The listing builds one solid part. Answer for the finished solid, in the listing's coordinates (mm). A direction names the side the tool comes from. Give positions to 0.01 mm unless a question says otherwise; leave off trailing zeros. Write each loop counter-clockwise with the first axis right and the second up, starting at its lowest first coordinate (ties: lowest second). Pieces come first, ordered by that corner, then holes. Notation, with made-up numbers: (-3.5, -20) - (9.5, -20) arc R28 ccw to (9.5, 16) - close; hole circle Ø5 at (31, 57.5). An arc over 180 degrees is marked (long way). Answer in a Markdown table with one row per item. Add a question column.
from build123d import *

# Parameters (mm, degrees)
SKIZZE1_W                       = 100
SKIZZE1_H                       = 50
AUFSATZ_LINEAR_AUSTRAGEN2_DEPTH = 25
SKIZZE4_R                       = 10
SCHNITT_LINEAR_AUSTRAGEN3_DEPTH = 115.564392374
SKIZZE5_W                       = 90
SKIZZE5_H                       = 40
SCHNITT_LINEAR_AUSTRAGEN4_DEPTH = 10
SKIZZE7_W                       = 25
SKIZZE7_H                       = 40
SCHNITT_LINEAR_AUSTRAGEN5_DEPTH = 10
VERRUNDUNG1_R                   = 10
VERRUNDUNG2_R                   = 10
SKIZZE8_W                       = 2
SKIZZE8_H                       = 40
SCHNITT_LINEAR_AUSTRAGEN6_DEPTH = 10
VERRUNDUNG3_R                   = 10


with BuildPart() as part:
    # Skizze1 → Aufsatz-Linear austragen2 (new body)
    with BuildSketch(Plane.XY):
        with Locations((50, 25)):
            Rectangle(SKIZZE1_W, SKIZZE1_H)
    extrude(amount=AUFSATZ_LINEAR_AUSTRAGEN2_DEPTH)

    # Skizze4 → Schnitt-Linear austragen3 (cut, through all)
    with BuildSketch(Plane(origin=(0, 50, 0), x_dir=(1, 0, 0), z_dir=(0, 1, 0))):
        with Locations((20, -25)):
            Circle(SKIZZE4_R)
        with Locations((80, -25)):
            Circle(SKIZZE4_R)
    extrude(amount=-SCHNITT_LINEAR_AUSTRAGEN3_DEPTH, mode=Mode.SUBTRACT)

    # Skizze5 → Schnitt-Linear austragen4 (cut)
    with BuildSketch(Plane(origin=(0, 0, 0), x_dir=(-1, 0, 0), z_dir=(0, 0, -1))):
        with Locations((-50, 25)):
            Rectangle(SKIZZE5_W, SKIZZE5_H)
    extrude(amount=-SCHNITT_LINEAR_AUSTRAGEN4_DEPTH, mode=Mode.SUBTRACT)

    # Skizze7 → Schnitt-Linear austragen5 (cut)
    with BuildSketch(Plane(origin=(0, 0, 10), x_dir=(-1, 0, 0), z_dir=(0, 0, -1))):
        with Locations((-50, 25)):
            Rectangle(SKIZZE7_W, SKIZZE7_H)
    extrude(amount=-SCHNITT_LINEAR_AUSTRAGEN5_DEPTH, mode=Mode.SUBTRACT)

    # Verrundung1
    verrundung1_edges = [part.edges().sort_by_distance(p)[0] for p in [
        (37.5, 25, 10),
    ]]
    fillet(verrundung1_edges, radius=VERRUNDUNG1_R - 0.0001)  # a hair under: the kernel refuses the full size

    # Verrundung2
    verrundung2_edges = [part.edges().sort_by_distance(p)[0] for p in [
        (62.5, 25, 10),
    ]]
    fillet(verrundung2_edges, radius=VERRUNDUNG2_R - 0.0001)  # a hair under: the kernel refuses the full size

    # Skizze8 → Schnitt-Linear austragen6 (cut)
    with BuildSketch(Plane(origin=(0, 0, 10), x_dir=(-1, 0, 0), z_dir=(0, 0, -1))):
        with Locations((-94, 25)):
            Rectangle(SKIZZE8_W, SKIZZE8_H)
    extrude(amount=-SCHNITT_LINEAR_AUSTRAGEN6_DEPTH, mode=Mode.SUBTRACT)

    # Verrundung3
    verrundung3_edges = [part.edges().sort_by_distance(p)[0] for p in [
        (93, 25, 10),
    ]]
    fillet(verrundung3_edges, radius=VERRUNDUNG3_R - 0.0001)  # a hair under: the kernel refuses the full size


solid = part.part
1. Straight lines are drawn through the part: L1, parallel to X at y = 8, z = 9.75; L2, parallel to Y at x = 33.5, z = 10.75; L3, parallel to X at y = 43.5, z = 20.25. For each, find the intervals that lie inside material, in ascending order. Write a range as [from, to].
2. A tool of negligible diameter and unlimited length cuts with its end or side. For faces 1 (the face through (20, 25, 15)), 2 (the face through (51, 45, 8)), from which of +Z, -Z, +X, -X, +Y, -Y can it reach the whole face along a straight path? Write none if from no direction.
3. Given pin 1 Ø10 at (x, z) = (33, 5.5) entering from -Y; pin 2 Ø8.5 at (x, y) = (75, 18.5) entering from -Z; pin 3 Ø7.5 at (x, y) = (56, 16) entering from -Z, each flat-ended and moving along its own axis, determine where each tip first touches the part or whether it passes through.
4. Section B-B (z = 7.5) is taken. Give the vertices of the cut face in (x, y).
5. The mould has two halves that part along X. Classify faces 3 (the face through (78, 25, 10)), 4 (the face through (46.1, 4.7, 0)), 5 (the face through (0, 25, 12)): +X half, -X half, draft (parallel to the pull), parting line (faces both ways), or undercut.
6. Section D-D (x = 86) is taken. Give the vertices of the cut face in (y, z).
7. Section C-C (z = 13.25) is taken. Give the vertices of the cut face in (x, y), and give its area (3 significant figures).
Geometry check:
| question | item | result |
|---|---|---|
| 1 | L1 | [0, 5], [95, 100] |
| 1 | L2 | [0, 5], [45, 50] |
| 1 | L3 | [0, 11.2], [28.8, 71.2], [88.8, 100] |
| 2 | face 1 | +Z, +Y, -Y |
| 2 | face 2 | -Z |
| 3 | pin 1 | y = 0 |
| 3 | pin 2 | z = 10 |
| 3 | pin 3 | z = 20 |
| 4 | outline | (0, 0) - (100, 0) - (100, 50) - (0, 50) - close; hole (5, 5) - (95, 5) - (95, 45) - (5, 45) - close |
| 5 | face 3 | undercut |
| 5 | face 4 | draft |
| 5 | face 5 | -X half |
| 6 | outline | (0, 0) - (5, 0) - (5, 10.46) - (45, 10.46) - (45, 0) - (50, 0) - (50, 17) - (0, 17) - close |
| 7 | outline | (0, 0) - (100, 0) - (100, 50) - (0, 50) - close; hole (34.88, 5) - (65.12, 5) - (65.12, 45) - (34.88, 45) - close; hole (90.38, 5) - (95, 5) - (95, 45) - (90.38, 45) - close |
| 7 | area | 3,610 mm² |
